The listing builds one solid part. Answer for the finished solid, in the listing's coordinates (mm). Give positions to 0.01 mm unless a question says otherwise; leave off trailing zeros. Write each loop counter-clockwise with the first axis right and the second up, starting at its lowest first coordinate (ties: lowest second). Pieces come first, ordered by that corner, then holes. Notation, with made-up numbers: M 28,-29.75 L 65,-29.75 A31 ccw 65,6.25 Z; hole C 38.25,1 d1. An arc over 180 degrees is marked long. Return JSON: item names as keys, results as strings.
Autodesk Inventor part; units mm, degrees
ref_plane "YZ Plane" through (0, 0, 0) normal (1, 0, 0) x (0, 1, 0)
ref_plane "XZ Plane" through (0, 0, 0) normal (0, 1, 0) x (-1, 0, 0)
ref_plane "XY Plane" through (0, 0, 0) normal (0, 0, 1) x (1, 0, 0)
sketch "Sketch1" plane through (0, 0, 0) normal (0, 0, 1) x (1, 0, 0)
  line L0 (0, 0) -> (491.0582, 0)
  line L1 (491.0582, 0) -> (491.0582, 508)
  line L2 (491.0582, 508) -> (0, 508)
  line L3 (0, 508) -> (0, 0)
  dimension "d0" = 491.0582
  dimension "d1" = 508
extrude "Extrusion1" add sketch "Sketch1" along normal blind 3.175
sketch "Sketch2" plane through (0, 0, 3.175) normal (0, 0, 1) x (1, 0, 0)
  line L0 (29.6291, 469.9) -> (461.4291, 469.9)
  line L1 (461.4291, 469.9) -> (461.4291, 38.1)
  line L2 (461.4291, 38.1) -> (29.6291, 38.1)
  line L3 (29.6291, 38.1) -> (29.6291, 469.9)
  line L4 (245.5291, 38.1) -> (245.5291, 0)
  line L5 (0, 0) -> (491.0582, 0)
  line L6 (245.5291, 469.9) -> (245.5291, 508)
  line L7 (491.0582, 508) -> (0, 508)
  line L8 (29.6291, 254) -> (0, 254)
  line L9 (0, 508) -> (0, 0)
  line L10 (461.4291, 254) -> (491.0582, 254)
  line L11 (491.0582, 0) -> (491.0582, 508)
  dimension "d4" = 431.8
  dimension "d5" = 431.8
extrude "Extrusion2" cut sketch "Sketch2" against normal blind 3.175 contours L0 L1 L2 L3
properties part number "window outer"
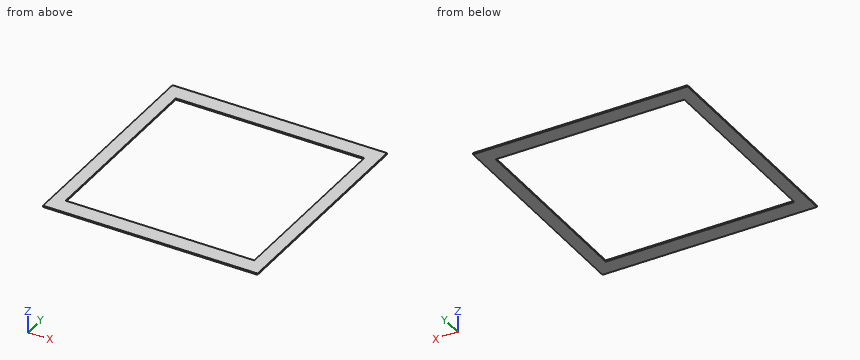
Item 1: Find the intervals of material crossed by line 1 (X direction, y = 360.5, z = 2.25); line 2 (Y direction, x = 259, z = 1.25), in increasing order.
Geometry results:
{"line 1": "x = 0 to 29.63, 461.43 to 491.06", "line 2": "y = 0 to 38.1, 469.9 to 508"}
Item 2: A cutting plane is placed at B-B, the plane z = 2.5. Write down the section's boundary in (x, y), plus the area to 3 significant figures.
Geometry results:
{"outline": "M 0,0 L 491.06,0 L 491.06,508 L 0,508 Z; hole M 29.63,38.1 L 461.43,38.1 L 461.43,469.9 L 29.63,469.9 Z", "area": "63,000 mm2"}
Item 3: A cutting plane is placed at A-A, the plane y = 187. Write down the section's boundary in (x, z) (3 decimals), plus the area to 3 significant figures.
Geometry results:
{"outline": "M 0,0 L 29.629,0 L 29.629,3.175 L 0,3.175 Z; M 461.429,0 L 491.058,0 L 491.058,3.175 L 461.429,3.175 Z", "area": "188 mm2"}
Item 4: A cutting plane is placed at C-C, the plane x = 436.5. Write down the section's boundary in (y, z) (3 decimals), plus the area to 3 significant figures.
Geometry results:
{"outline": "M 0,0 L 38.1,0 L 38.1,3.175 L 0,3.175 Z; M 469.9,0 L 508,0 L 508,3.175 L 469.9,3.175 Z", "area": "242 mm2"}
